Can you work these out from the model? Positions are in its coordinate system, mm. Round coordinates to 2 decimals unless told otherwise and drop trailing zeros. Write each loop counter-clockwise with the first axis right and the second up, starting at its lowest first coordinate (ties: lowest second). Pieces come first, ordered by that corner, then holes. Notation, with made-up numbers: M -4.75,40 L 39.25,40 A22 cw 39.25,68 Z; hole C 68,-3.5 d4. An arc over 180 degrees is marked long. Use one line per item in the form item = value. Start each with the question number.
```python
from build123d import *

# Parameters (mm, degrees)
F1_DEPTH  = 3
F2_COUNT  = 11
F3_R      = 7
F4_DEPTH  = 10
F5_R      = 3
F6_DEPTH  = 13.001
F7_R      = 2
F8_DEPTH  = 11.410776
F9_R      = 2
F10_DEPTH = 11.410776


with BuildPart() as f1:
    # F0 (on Right) → F1 (new body)
    with BuildSketch(Plane.YZ):
        with BuildLine():
            add(Edge.make_bspline(
                [(2.394727, 8.15569), (1.48914, 8.651781), (0.734067, 9.406854), (0.200703, 11.498248)],
                knots=[0, 0, 0, 0, 3.998304, 3.998304, 3.998304, 3.998304], degree=3))
            ThreePointArc((0.200703, 11.498248), (0, 11.5), (-0.200703, 11.498248))
            add(Edge.make_bspline(
                [(-2.394727, 8.15569), (-1.48914, 8.651781), (-0.734067, 9.406854), (-0.200703, 11.498248)],
                knots=[0, 0, 0, 0, 3.998304, 3.998304, 3.998304, 3.998304], degree=3))
            Line((-2.394727, 8.15569), (0, 0))
            Line((0, 0), (2.394727, 8.15569))
        make_face()
    extrude(amount=F1_DEPTH)

    # F2: F1 ×11 about axis
    f2_axis = Axis((1.5, 0, 0), (1, 0, 0))


with BuildPart() as f1_1:
    add(f1.part)
    for i in range(1, F2_COUNT):
        add(f1.part.rotate(f2_axis, i * 360 / F2_COUNT))

    # F3 (on face) → F4 (join)
    with BuildSketch(Plane(origin=(0, 0, 0), x_dir=(0, -1, 0), z_dir=(-1, 0, 0))):
        Circle(F3_R)
    extrude(amount=F4_DEPTH)

    # F5 (on face) → F6 (cut, through all)
    with BuildSketch(Plane(origin=(-10, 0, 0), x_dir=(0, -1, 0), z_dir=(-1, 0, 0))):
        Circle(F5_R)
    extrude(amount=-F6_DEPTH, mode=Mode.SUBTRACT)

    # F7 (on Front) → F8 (cut, through all)
    with BuildSketch(Plane.XZ):
        with Locations((-5, 0)):
            Circle(F7_R)
    extrude(amount=-F8_DEPTH, mode=Mode.SUBTRACT)

    # F9 (on Front) → F10 (cut, through all)
    with BuildSketch(Plane.XZ):
        with Locations((-5, 0)):
            Circle(F9_R)
    extrude(amount=F10_DEPTH, mode=Mode.SUBTRACT)


solid = f1_1.part
```
1. If we section it at C-C (x = -8.5): List the corners of the cut face in (y, z) for me, and give its area (3 significant figures).
2. If we section it at A-A (x = -5): List the corners of the cut face in (y, z) for me.
3. Please list where these lines run through material, in increasing order: line 1 along Z through (x, y) = (-2.75, 0); line 2 along Y through (x, z) = (-0.25, 0.25); line 3 along X through (y, z) = (-8.5, -0.5).
4. Will these pins go through, and if not, where does the flat tip stop? pin 1 (4.5 mm diameter, centred on x = -5, z = 0, fed in from -Y); pin 2 (1 mm diameter, centred on y = -2, z = -7.5, fed in from -X); pin 3 (11.5 mm diameter, centred on y = -2, z = 1.5, fed in from -X); pin 4 (1.5 mm diameter, centred on x = -8.5, z = -7, fed in from +Y).
5. If we mould it in two halves opening along Z, with no side actions, what happens to faces 1 (the face through (-4.93, -6.466, -2.681)), 2 (the face through (-3.153, 4.585, -0.766)), 3 (the face through (0, 2, 7))? For each: pulls with the +Z half, pulls with the -Z half, needs draft (parallel to the pull), parting line crosses it, or undercut.
6. If we section it at B-B (z = -1): State how many separate pieces and enclosed holes the cut face has, and give its area (3 significant figures).
Model answer:
q1.outline = C 0,0 d14; hole C 0,0 d6
q1.area = 126 mm2
q2.outline = M -6.71,-2 A7 ccw 6.71,-2 L 2.24,-2 A3 cw -2.24,-2 Z; M -6.71,2 L -2.24,2 A3 cw 2.24,2 L 6.71,2 A7 ccw Z
q3.line_1 = -7 to -3, 3 to 7
q3.line_2 = -7 to -2.99, 2.99 to 7
q3.line_3 = 0 to 3
q4.pin_1 = -7
q4.pin_2 = 0
q4.pin_3 = -10
q4.pin_4 = 3.15
q5.face_1 = parting line crosses it
q5.face_2 = undercut
q5.face_3 = needs draft
q6.separate_pieces = 4
q6.enclosed_holes = 0
q6.area = 99.5 mm2
